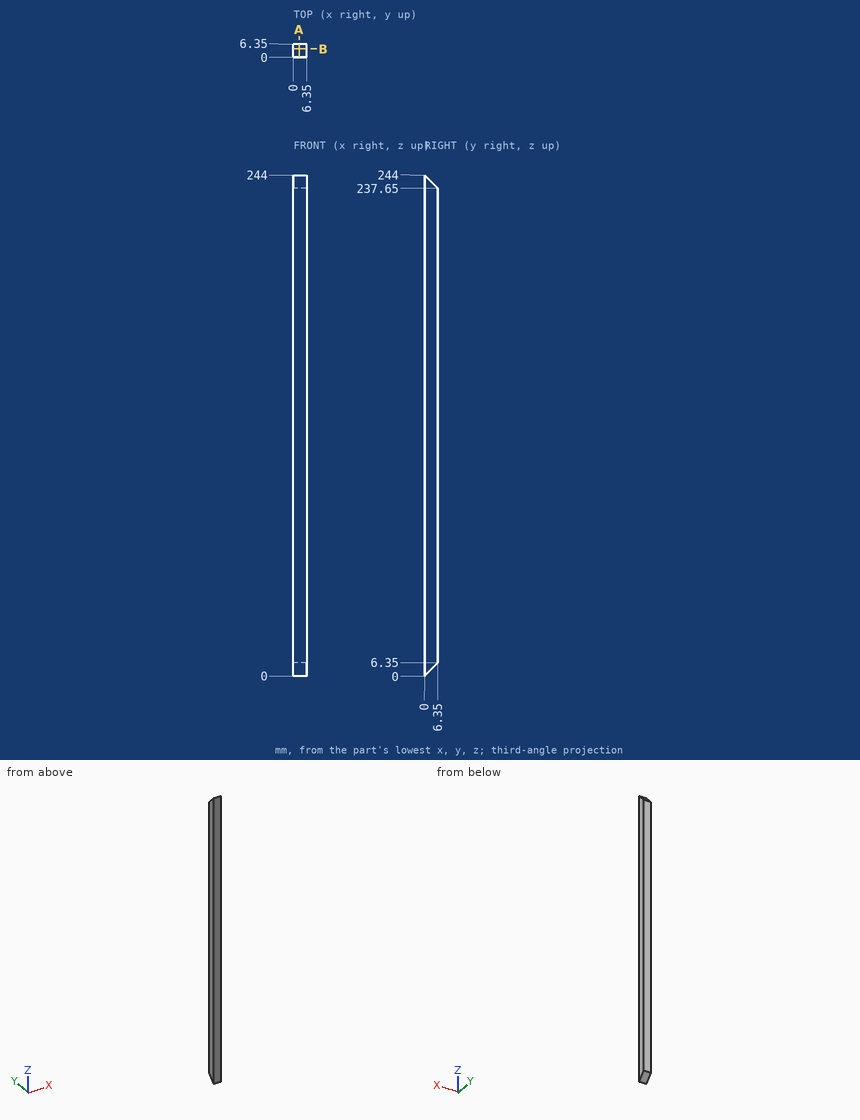
Drawing for the job (mm, zero at the part's lowest x, y, z). Give positions to 0.01 mm unless a question says otherwise; leave off trailing zeros. Loops run counter-clockwise (first coordinate to the right, second up) from the corner with the lowest first, then second, coordinate; pieces in that order, holes last. Notation, with made-up numbers: (34, -33.75) - (81, -33.75) arc R26 cw to (81, -1.75) - close; hole circle Ø8 at (65, 56.5). An arc over 180 degrees is marked (long way). Write item = value, one per line. Start each with the question number.
1) Drop flat-ended pins along their axis: pin 1 Ø3 at (x, y) = (3.5, 1) entering from +Z; pin 2 Ø2 at (x, y) = (3, 4.5) entering from +Z. Give the stop position or say it passes through.
2) Probe probe 1 along Z at (x, y) = (4.75, 3.75); probe 2 along Z at (x, y) = (2.75, 4.5). List the from-to ranges inside material, lowest first. Write a range as from..to.
3) Band-saw the part on B-B on y = 4. Give the cut face in (x, z).
4) Band-saw the part on A-A on x = 2.75. Give the cut face in (y, z).
Final values:
q1.pin_1 = 244
q1.pin_2 = 240.5
q2.probe_1 = 3.75..240.25
q2.probe_2 = 4.5..239.5
q3.outline = (0, 4) - (6.35, 4) - (6.35, 240) - (0, 240) - close
q4.outline = (0, 0) - (6.35, 6.35) - (6.35, 237.65) - (0, 244) - close
